Source: CAD feature listing. Evaluate the final solid. Frame: model axes, mm. A direction names the side the tool comes from. Give positions to 0.01 mm unless a question says otherwise; leave off trailing zeros. Loops run counter-clockwise (first coordinate to the right, second up) from the corner with the lowest first, then second, coordinate; pieces in that order, holes last.
Autodesk Inventor part; units mm, degrees
ref_plane "YZ Plane" through (0, 0, 0) normal (1, 0, 0) x (0, 1, 0)
ref_plane "XZ Plane" through (0, 0, 0) normal (0, 1, 0) x (-1, 0, 0)
ref_plane "XY Plane" through (0, 0, 0) normal (0, 0, 1) x (1, 0, 0)
sketch "草圖1" plane through (0, 0, 0) normal (0, 1, 0) x (-1, 0, 0)
  line L0 (-33.5, 27) -> (33.5, 27)
  line L1 (33.5, 27) -> (33.5, -27)
  line L2 (33.5, -27) -> (-33.5, -27)
  line L3 (-33.5, -27) -> (-33.5, 27)
  line L4 (-33.5, 27) -> (33.5, -27) construction
  line L5 (33.5, 27) -> (-33.5, -27) construction
  line L6 (43.5, -4.5) -> (33.5, -4.5)
  line L7 (33.5, -4.5) -> (33.5, 4.5)
  line L8 (33.5, 4.5) -> (43.5, 4.5)
  line L9 (43.5, 4.5) -> (43.5, -4.5)
  line L10 (-33.5, -4.5) -> (-43.5, -4.5)
  line L11 (-43.5, -4.5) -> (-43.5, 4.5)
  line L12 (-43.5, 4.5) -> (-33.5, 4.5)
  line L13 (-33.5, 4.5) -> (-33.5, -4.5)
  point P0 (0, 0)
  point P1 (33.5, 0)
  point P2 (-33.5, 0)
  point P3 (-33.5, 4.5)
  point P4 (-33.5, -4.5)
  dimension "d0" = 67
  dimension "d1" = 54
  dimension "d2" = 9
  dimension "d3" = 10
extrude "擠出1" add sketch "草圖1" along normal blind 250
sketch "草圖2" plane through (-33.5, 0, 27) normal (0, 0, 1) x (1, 0, 0)
  circle A0 centre (33.5, 102) radius 30
  line L0 (0, 0) -> (67, 0)
  line L1 (3.5, 102) -> (63.5, 102)
  line L2 (63.5, 102) -> (63.5, -30.9469)
  line L3 (63.5, -30.9469) -> (3.5, -30.9469)
  line L4 (3.5, -30.9469) -> (3.5, 102)
  point P0 (33.5, 0)
  point P1 (33.5, 0)
  point P2 (63.5, 102)
  dimension "d6" = 102
  dimension "d7" = 60
extrude "擠出2" cut sketch "草圖2" against normal through all
sketch "草圖3" plane through (-33.5, 250, 27) normal (0, 0, 1) x (1, 0, 0)
  line L0 (-69.9684, -200) -> (136.9684, -200)
  line L1 (136.9684, -200) -> (136.9684, -250)
  line L2 (136.9684, -250) -> (-69.9684, -250)
  line L3 (-69.9684, -250) -> (-69.9684, -200)
  point P0 (33.5, -250)
  point P1 (33.5, -250)
  dimension "d10" = 50
extrude "擠出3" cut sketch "草圖3" against normal through all
sketch "草圖4" plane through (33.5, 250, -27) normal (0, 0, -1) x (-1, 0, 0)
  arc A0 (63.5, -148) -> (3.5, -148) centre (33.5, -148) ccw construction
  circle A1 centre (33.5, -136) radius 30
  line L0 (63.5, -200) -> (3.5, -200)
  line L1 (3.5, -200) -> (3.5, -136)
  line L2 (3.5, -136) -> (63.5, -136)
  line L3 (63.5, -136) -> (63.5, -200)
  point P0 (33.5, -250)
  point P1 (63.5, -200)
  dimension "d13" = 12
  dimension "d14" = 60
sketch "草圖5" plane through (-33.5, 250, 27) normal (0, 0, 1) x (1, 0, 0)
  circle A0 centre (33.5, -134) radius 30
  arc A1 (63.5, -148) -> (3.5, -148) centre (33.5, -148) ccw construction
  line L0 (63.5, -200) -> (3.5, -200)
  line L1 (3.5, -200) -> (3.5, -134)
  line L2 (3.5, -134) -> (63.5, -134)
  line L3 (63.5, -134) -> (63.5, -200)
  point P0 (33.5, -250)
  dimension "d15" = 14
  dimension "d16" = 60
loft "斷面混成1" cut profiles "草圖4", "草圖5"
properties part number "Slider-4"
(1) Section A-A, the plane y = 100.5. Return the cut outline in (x, z).
A:
outline: (-43.5, -4.5) - (-33.5, -4.5) - (-33.5, -27) - (-30, -27) - (-30, 27) - (-33.5, 27) - (-33.5, 4.5) - (-43.5, 4.5) - close; (30, -27) - (33.5, -27) - (33.5, -4.5) - (43.5, -4.5) - (43.5, 4.5) - (33.5, 4.5) - (33.5, 27) - (30, 27) - close
(2) Mould query, pull axis X, two halves, no side actions, for faces 5 (the flat face through (-30, 83, 0)), 6 (the flat face through (39, 149, 4.5)), 7 (the flat face through (30, 83, 0)), 8 (the flat face through (-43.5, 149, 0)). Classes: pulls with the +X half, pulls with the -X half, needs draft (parallel to the pull), parting line crosses it, or undercut.
A:
face 5: undercut
face 6: needs draft
face 7: undercut
face 8: pulls with the -X half
(3) Section B-B, the plane y = 212. Return the cut outline in (x, z).
A:
outline: (-43.5, -4.5) - (-33.5, -4.5) - (-33.5, -27) - (33.5, -27) - (33.5, -4.5) - (43.5, -4.5) - (43.5, 4.5) - (33.5, 4.5) - (33.5, 27) - (-33.5, 27) - (-33.5, 4.5) - (-43.5, 4.5) - close
(4) Reachability of faces 1 (the flat face through (38, 149, -4.5)), 2 (the flat face through (-38, 149, 4.5)), 3 (the flat face through (-33.5, 149, -16)), 4 (the flat face through (33.5, 149, 16)) from +Z, -Z, +X, -X, +Y, -Y: full face, straight path, thin tool, end or side. Return the list, or none.
A:
face 1: -Z, +X, +Y, -Y
face 2: +Z, -X, +Y, -Y
face 3: -Z, -X, +Y, -Y
face 4: +Z, +X, +Y, -Y
(5) First-contact query: pin 1 (5 mm diameter, centred on x = -40, y = 172, fed in from -Z); pin 2 (6 mm diameter, centred on y = 81, z = -15, fed in from -X); pin 3 (3 mm diameter, centred on x = 40, y = 138, fed in from +Z). Flat tips, straight axial feed; report the tip coordinate or a pass-through.
A:
pin 1: stops at z = -4.5
pin 2: stops at x = -33.5
pin 3: stops at z = 4.5
(6) Ray query, line 1 along X through (y, z) = (112.5, 2); line 2 along X through (y, z) = (64, -17.5); line 3 along X through (y, z) = (232.5, -6.5). Return the intervals inside material, ascending.
A:
line 1: x = -43.5 to -30, 30 to 43.5
line 2: x = -33.5 to -30, 30 to 33.5
line 3: x = -33.5 to 33.5
